Autodesk Inventor part; units mm, degrees
ref_plane "YZ Plane" through (0, 0, 0) normal (1, 0, 0) x (0, 1, 0)
ref_plane "XZ Plane" through (0, 0, 0) normal (0, 1, 0) x (-1, 0, 0)
ref_plane "XY Plane" through (0, 0, 0) normal (0, 0, 1) x (1, 0, 0)
sketch "Skizze1" plane through (0, 0, 0) normal (0, 0, 1) x (1, 0, 0)
  line L0 (-10, -10) -> (10, -10)
  line L1 (10, -10) -> (10, 10)
  line L2 (10, 10) -> (-10, 10)
  line L3 (-10, 10) -> (-10, -10)
  line L4 (-10, -10) -> (10, 10) construction
  line L5 (10, -10) -> (-10, 10) construction
  point P0 (0, 0)
  dimension "d0" = 20
  dimension "d1" = 20
extrude "Extrusion1" add sketch "Skizze1" along normal blind 2
sketch "Skizze2" plane through (0, 0, 2) normal (0, 0, 1) x (1, 0, 0)
  circle A0 centre (0, 0) radius 5
  dimension "d4" = 10
extrude "Extrusion2" add sketch "Skizze2" along normal blind 20
sketch "Skizze3" plane through (0, 0, 2) normal (0, 0, 1) x (1, 0, 0)
  line L0 (10, 10) -> (-10, 10)
  line L1 (-10, 10) -> (-10, -10)
  line L2 (10, -10) -> (10, 10)
  line L3 (-10, -10) -> (10, -10)
  point P0 (0, 0)
  point P1 (-6, 6)
  point P2 (6, 6)
  point P3 (6, -6)
  point P4 (-6, -6)
  dimension "d7" = 4
  dimension "d8" = 4
  dimension "d9" = 4
  dimension "d10" = 4
  dimension "d11" = 4
  dimension "d12" = 4
  dimension "d13" = 4
  dimension "d14" = 4
hole "Bohrung1" at (-6, 6, 2) at (6, 6, 2) at (6, -6, 2) at (-6, -6, 2) direction (0, 0, -1) diameter 2.95 end through all
properties part number "Laserhalter Mittelteil 29112018"
The listing builds one solid part. Answer for the finished solid, in the listing's coordinates (mm). A direction names the side the tool comes from. Round coordinates to 2 decimals unless told otherwise and drop trailing zeros. Write each loop counter-clockwise with the first axis right and the second up, starting at its lowest first coordinate (ties: lowest second). Pieces come first, ordered by that corner, then holes. Notation, with made-up numbers: M 64,0 L 83,0 A9 cw 83,8 Z; hole C 21,18.25 d11. An arc over 180 degrees is marked long. Write each question's results on one line, items separated by ' | '. Start each with the question number.
(1) Determine the mould class of faces 3 (the flat face through (-10, 0, 1)), 4 (the cylindrical face through (-6.065, -4.526, 0.986)), 5 (the flat face through (10, 0, 1)) for opening direction X: +X half, -X half, draft (parallel to the pull), parting line (faces both ways), or undercut.
(2) Each of these flat-tipped pins is pushed along its axis until it touches: P1, Ø10, axis at x = -7.5, z = 16.5, coming from the -Y side; P2, Ø12, axis at x = 2, z = 17.5, coming from the -Y side; P3, Ø1, axis at x = 1, y = 6, coming from the +Z side. Where does it stop, or does it pass through?
(3) The part is cut by section A-A, the plane y = 6. Write down the section's boundary in (x, z) (3 decimals), and give its area (3 significant figures).
(4) The part is cut by section C-C, the plane y = 0. Write down the section's boundary in (x, z), and give its area (3 significant figures).
(5) Find the intervals of material crossed by line 1 (Y direction, x = -6, z = 1.25) (3 decimals); line 2 (Z direction, x = -6.5, y = 2.25), in increasing order.
(6) For faces 1 (the cylindrical face through (-1.08, 4.88, 11.86)), 2 (the flat face through (0, 10, 1)), determine the directions among +Z, -Z, +X, -X, +Y, -Y from which every point of the face is accessible in a straight line to the end or side of a thin tool.
Worked answers:
1) face 3: -X half | face 4: undercut | face 5: +X half
2) P1: stops at y = -4.33 | P2: stops at y = -5 | P3: stops at z = 2
3) outline: M -10,0 L -7.475,0 L -7.475,2 L -10,2 Z; M -4.525,0 L 4.525,0 L 4.525,2 L -4.525,2 Z; M 7.475,0 L 10,0 L 10,2 L 7.475,2 Z | area: 28.2 mm²
4) outline: M -10,0 L 10,0 L 10,2 L 5,2 L 5,22 L -5,22 L -5,2 L -10,2 Z | area: 240 mm²
5) line 1: y = -10 to -7.475, -4.525 to 4.525, 7.475 to 10 | line 2: z = 0 to 2
6) face 1: +Z | face 2: +Z, -Z, +X, -X, +Y
